Here's how the part is built. I have some questions about the finished solid (model axes, mm). Face numbers are marked on the shaded views. A direction names the side the tool comes from. Give positions to 0.01 mm unless a question says otherwise; leave off trailing zeros. Order: outer loops, then holes, each group sorted by start corner. A loop starts at its lowest first (then second) coordinate and runs counter-clockwise, first axis right, second up. Notation, with made-up numbers: (61, 83.25) -> (72, 83.25) arc R16 ccw to (72, 95.25) -> close; hole circle Ø11 at (19.5, -7.5). An arc over 180 degrees is marked (long way). Write each question's results on one line, items separated by ' | '. Start each with the question number.
Q1. Imagine slicing it at A-A, the plane y = 10. Please give me the cut outline in (x, z).
Q2. I'm going to push flat-ended pins straight in: pin 1 (15 mm diameter, centred on x = 30.5, z = 39, fed in from -Y); pin 2 (12 mm diameter, centred on x = -24.5, y = 65, fed in from +Z); pin 3 (12 mm diameter, centred on y = 51.5, z = 25, fed in from -X); pin 4 (10 mm diameter, centred on y = -3, z = 14.5, fed in from +X). Where does each tip first touch, or does it pass through?
Q3. For the marked faces 1, 2 and 3, which set-ups out of +Z, -Z, +X, -X, +Y, -Y let a thin tool reach every point of the face, with its end or its side?
Q4. Imagine slicing it at C-C, the plane x = -17.5. Please give me the cut outline in (y, z), then the cut area to 3 significant figures.
Q5. I need wall thicknesses on line 1 along Z through (x, y) = (-12.5, 53.5); line 2 along X through (y, z) = (4, 3); line 3 along Y through (x, z) = (21.5, 15.5). Which ranges of each line are inside material? Lowest first, please. Write a range as [from, to].
Q6. Imagine slicing it at D-D, the plane x = 4.5. Please give me the cut outline in (y, z), then the cut area to 3 significant figures.
Q7. Thinking about a two-plate mould opening in X: for the marked faces 4, 5, 6 and 7, which applies, pulls with the +X half, pulls with the -X half, needs draft (parallel to the pull), parting line crosses it, or undercut?
Q8. Imagine slicing it at B-B, the plane z = 10. Please give me the cut outline in (x, y), then the cut area to 3 significant figures.
```python
from build123d import *

# Parameters (mm, degrees)
F1_DEPTH = 50
F2_R     = 7.4
F2_R_2   = 3
F3_DEPTH = 28
F4_W     = 2
F4_H     = 27.5
F5_DEPTH = 33
F7_DEPTH = 2
F9_DEPTH = 25


with BuildPart() as f1:
    # F0 (on Right) → F1 (new body)
    with BuildSketch(Plane.YZ):
        with BuildLine():
            ThreePointArc((0, 5), (1.464466, 1.464466), (5, 0))
            Line((5, 0), (70.5, 0))
            ThreePointArc((70.5, 0), (74.035534, 1.464466), (75.5, 5))
            Line((75.5, 5), (75.5, 55.5))
            ThreePointArc((75.5, 55.5), (74.035534, 59.035534), (70.5, 60.5))
            Line((70.5, 60.5), (5, 60.5))
            ThreePointArc((5, 60.5), (1.464466, 59.035534), (0, 55.5))
            Line((0, 55.5), (0, 5))
        make_face()
    extrude(amount=F1_DEPTH)

    # F2 (on face) → F3 (join)
    with BuildSketch(Plane(origin=(0, 0, 0), x_dir=(0, -1, 0), z_dir=(-1, 0, 0))):
        with Locations((-53.5, 27.5)):
            Circle(F2_R)
        with Locations((-53.5, 27.5)):
            Circle(F2_R_2, mode=Mode.SUBTRACT)
    extrude(amount=F3_DEPTH)

    # F4 (on face) → F5 (join)
    with BuildSketch(Plane(origin=(0, 0, 0), x_dir=(0, -1, 0), z_dir=(-1, 0, 0))):
        with Locations((-32.5, 13.75)):
            Rectangle(F4_W, F4_H)
    extrude(amount=F5_DEPTH)

    # F6 (on face) → F7 (join)
    with BuildSketch(Plane(origin=(-33, 0, 0), x_dir=(0, -1, 0), z_dir=(-1, 0, 0))):
        with BuildLine():
            Line((-33.5, 20), (-33.5, 0))
            Line((-33.5, 0), (13.5, 0))
            ThreePointArc((13.5, 0), (17.035534, 1.464466), (18.5, 5))
            Line((18.5, 5), (18.5, 15))
            ThreePointArc((18.5, 15), (17.035534, 18.535534), (13.5, 20))
            Line((13.5, 20), (-33.5, 20))
        make_face()
        with BuildLine():
            ThreePointArc((5.610631, 7.002041), (5.5, 7), (5.389369, 7.002041))
            Line((5.389369, 7.002041), (-20.389369, 7.002041))
            ThreePointArc((-20.389369, 7.002041), (-23.499577, 9.949607), (-20.490135, 12.999984))
            Line((-20.490135, 12.999984), (5.499998, 13))
            ThreePointArc((5.499998, 13), (8.49949, 10.055326), (5.610631, 7.002041))
        make_face(mode=Mode.SUBTRACT)
    extrude(amount=F7_DEPTH)

    # F8 (on face) → F9 (cut)
    with BuildSketch(Plane(origin=(0, 33.5, 0), x_dir=(-1, 0, 0), z_dir=(0, 1, 0))):
        Polygon((0, 27.5), (33, 20), (42.120021, 30.809933), (19.240811, 38.767923), align=None)
    extrude(amount=-F9_DEPTH, mode=Mode.SUBTRACT)


solid = f1.part
```
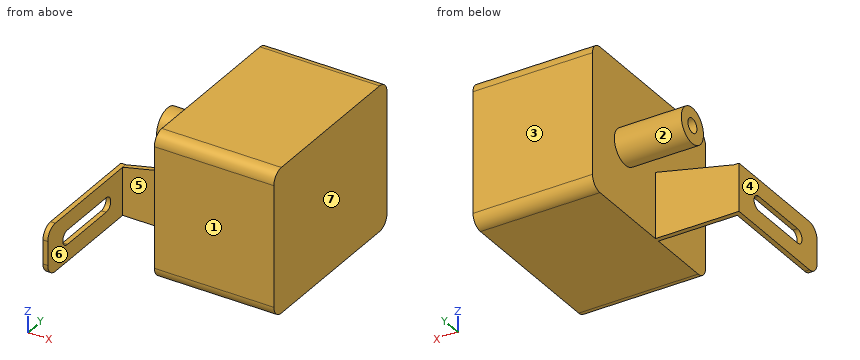
Geometry check:
1) outline: (-35, 0) -> (-33, 0) -> (-33, 7) -> (-35, 7) -> close; (-35, 13) -> (-33, 13) -> (-33, 20) -> (-35, 20) -> close; (0, 0) -> (50, 0) -> (50, 60.5) -> (0, 60.5) -> close
2) pin 1: y = 0 | pin 2: z = 32.45 | pin 3: x = -28 | pin 4: x = 50
3) face 1: +Z, -Z, +X, -Y | face 2: -X | face 3: +Z, -Z, +X, -X, +Y
4) outline: (31.5, 0) -> (33.5, 0) -> (33.5, 23.52) -> (31.5, 23.52) -> close; circle Ø14.8 at (53.5, 27.5); hole circle Ø6 at (53.5, 27.5) | area: 191 mm²
5) line 1: [20.1, 24.5], [30.5, 34.9] | line 2: [-35, -33], [0, 50] | line 3: [0, 75.5]
6) outline: (0, 5) arc R5 ccw to (5, 0) -> (70.5, 0) arc R5 ccw to (75.5, 5) -> (75.5, 55.5) arc R5 ccw to (70.5, 60.5) -> (5, 60.5) arc R5 ccw to (0, 55.5) -> close | area: 4,550 mm²
7) face 4: pulls with the -X half | face 5: undercut | face 6: undercut | face 7: pulls with the +X half
8) outline: (-35, -18.5) -> (-33, -18.5) -> (-33, -8.5) -> (-35, -8.5) -> close; (-35, 23.5) -> (-33, 23.5) -> (-33, 31.5) -> (0, 31.5) -> (0, 0) -> (50, 0) -> (50, 75.5) -> (0, 75.5) -> (0, 33.5) -> (-35, 33.5) -> close | area: 3,880 mm²
